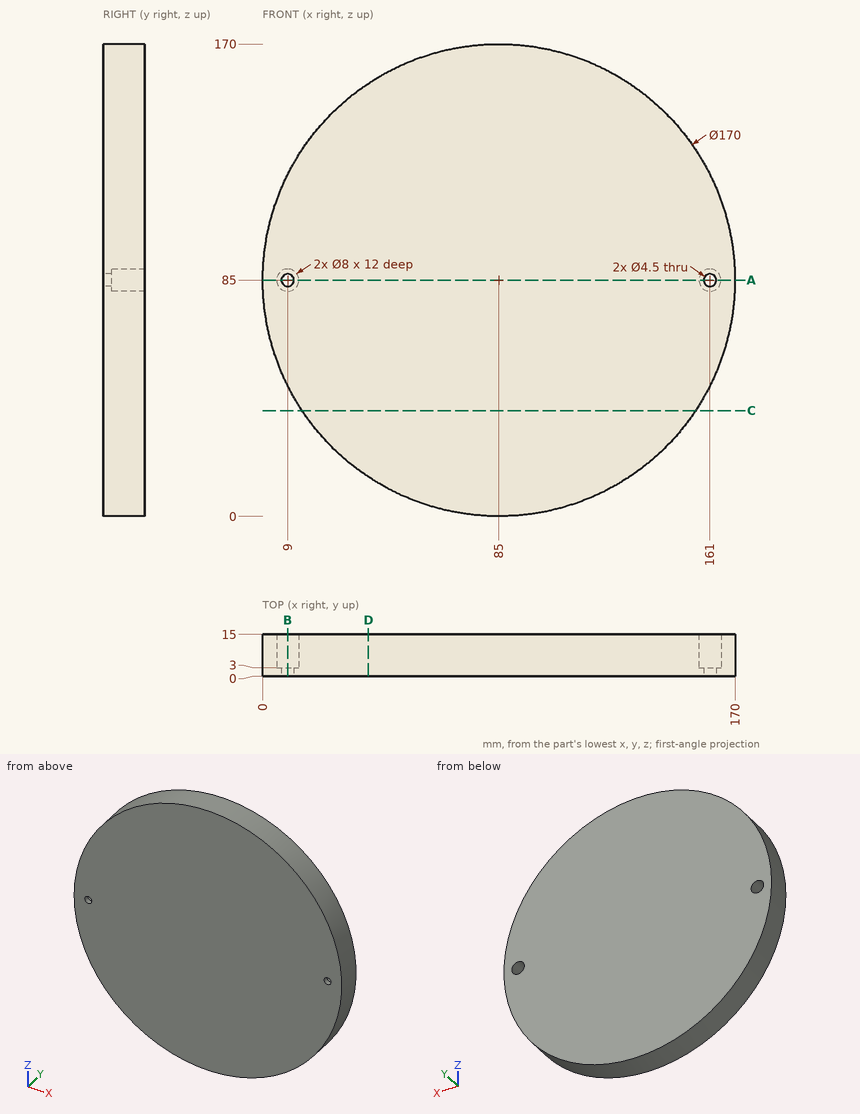
Can you work these out from the drawing? Everything is in mm from the part's minimum corner. Coordinates: 2 decimals unless noted, no trailing zeros. Write each loop counter-clockwise with the first axis right and the second up, starting at its lowest first coordinate (ties: lowest second). Pieces come first, ordered by that corner, then holes. Notation, with made-up numbers: (20.5, 81) -> (66.5, 81) arc R23 ccw to (66.5, 118) -> close; hole circle Ø2 at (12.5, -1). An arc over 180 degrees is marked (long way). Write each question's results on one line, items separated by ' | '. Start each with the question number.
Item 1: If we section it at C-C, the plane z = 38: Write out the boundary of the cut face in (x, y).
Item 2: If we section it at B-B, the plane x = 9: Write out the boundary of the cut face in (y, z), and give its area (3 significant figures).
Item 3: If we section it at D-D, the plane x = 38: Write out the boundary of the cut face in (y, z).
Item 4: I'm going to push flat-ended pins straight in: P1, Ø3, axis at x = 31.5, y = 8.5, coming from the +Z side; P2, Ø5, axis at y = 3.5, z = 73.5, coming from the +X side; P3, Ø1, axis at x = 27.5, y = 3, coming from the -Z side; P4, Ø3.5, axis at x = 9, z = 85, coming from the -Y side. Where does each tip first touch, or does it pass through?
Item 5: Please list where these lines run through material, in increasing order: probe 1 along Z at (x, y) = (9, 1.4); probe 2 along Z at (x, y) = (161.5, 14.5); probe 3 along Z at (x, y) = (115.5, 2.75).
Item 6: If we section it at A-A, the plane z = 85: Write out the boundary of the cut face in (x, y).
Answer block:
1) outline: (14.18, 0) -> (155.82, 0) -> (155.82, 15) -> (14.18, 15) -> close
2) outline: (0, 46.93) -> (15, 46.93) -> (15, 81) -> (3, 81) -> (3, 82.75) -> (0, 82.75) -> close; (0, 87.25) -> (3, 87.25) -> (3, 89) -> (15, 89) -> (15, 123.07) -> (0, 123.07) -> close | area: 1,030 mm²
3) outline: (0, 14.18) -> (15, 14.18) -> (15, 155.82) -> (0, 155.82) -> close
4) P1: z = 152.24 | P2: x = 169.52 | P3: z = 21.94 | P4: through
5) probe 1: 46.93 to 82.75, 87.25 to 123.07 | probe 2: 47.95 to 81.03, 88.97 to 122.05 | probe 3: 5.66 to 164.34
6) outline: (0, 0) -> (6.75, 0) -> (6.75, 3) -> (5, 3) -> (5, 15) -> (0, 15) -> close; (11.25, 0) -> (158.75, 0) -> (158.75, 3) -> (157, 3) -> (157, 15) -> (13, 15) -> (13, 3) -> (11.25, 3) -> close; (163.25, 0) -> (170, 0) -> (170, 15) -> (165, 15) -> (165, 3) -> (163.25, 3) -> close
